from build123d import *

# Parameters (mm, degrees)
BOSS_EXTRUDE1_DEPTH = 63.2
FILLET1_R           = 10
FILLET2_R           = 10
FILLET3_R           = 10
CUT_EXTRUDE1_REACH  = 139.674
SKETCH2_R           = 2.3
SKETCH3_R           = 1.75
CUT_EXTRUDE2_DEPTH  = 138.67396268
SKETCH4_R           = 3.25
CUT_EXTRUDE3_DEPTH  = 7


with BuildPart() as part:
    # Sketch1 → Boss-Extrude1 (new body)
    with BuildSketch(Plane.XY):
        Polygon((114.8, 0), (114.8, 22.5), (92.3, 22.5), (74.008186766, 22.5), (74.008186766, 26), (40.791813234, 26), (40.791813234, 22.5), (22.5, 22.5), (0, 22.5), (0, 0), (0, -16.2), (5, -16.2), (5, 0), (5, 17.5), (22.5, 17.5), (45.791813234, 17.5), (45.791813234, 21), (57.4, 21), (69.008186766, 21), (69.008186766, 17.5), (92.3, 17.5), (109.8, 17.5), (109.8, 0), (109.8, -16.2), (114.8, -16.2), align=None)
    extrude(amount=BOSS_EXTRUDE1_DEPTH)

    # Fillet1
    fillet1_edges = [part.edges().sort_by_distance(p)[0] for p in [
        (0, 22.5, 31.6),
        (114.8, 22.5, 31.6),
        (109.8, 17.5, 31.6),
        (5, 17.5, 31.6),
    ]]
    fillet(fillet1_edges, radius=FILLET1_R)

    # Fillet2
    # the kernel refuses this fillet: 10 mm, written as the material it takes off along each edge
    with BuildSketch(Plane(origin=(40.791813234, 26, -18.998355192), x_dir=(1, 0, 0), z_dir=(0, 0, 1))) as fillet2_piece_1:
        with BuildLine():
            CenterArc((7.599342077, -10), FILLET2_R, 90, 49.458398126)
            Line((0, -3.5), (-0.151986842, -3.37))
            ThreePointArc((-0.151986842, -3.37), (-0.2, -1.75), (-0.2, 0))
            Line((-0.2, 0), (0, 0.2))
            Line((0, 0.2), (7.599342077, 0.2))
            Line((7.599342077, 0.2), (7.599342077, 0))
        make_face()
    extrude(amount=101.196710384, mode=Mode.SUBTRACT)
    with BuildSketch(Plane(origin=(74.008186766, 26, -18.998355192), x_dir=(0, -1, 0), z_dir=(0, 0, 1))) as fillet2_piece_2:
        with BuildLine():
            CenterArc((10, -7.599342077), FILLET2_R, 130.541601874, 49.458398126)
            Line((0, -7.599342077), (-0.2, -7.599342077))
            Line((-0.2, -7.599342077), (-0.2, 0))
            Line((-0.2, 0), (0, 0.2))
            ThreePointArc((0, 0.2), (1.75, 0.2), (3.37, 0.151986842))
            Line((3.37, 0.151986842), (3.5, 0))
        make_face()
    extrude(amount=101.196710384, mode=Mode.SUBTRACT)

    # Fillet3
    # the kernel refuses this fillet: 10 mm, written as the material it takes off along each edge
    with BuildSketch(Plane(origin=(45.791813234, 17.5, -18.998355192), x_dir=(0, 1, 0), z_dir=(0, 0, 1))) as fillet3_piece_1:
        with BuildLine():
            CenterArc((10, 7.599342077), FILLET3_R, 180, 49.458398126)
            Line((0, 7.599342077), (-0.2, 7.599342077))
            Line((-0.2, 7.599342077), (-0.2, 0))
            Line((-0.2, 0), (0, -0.2))
            ThreePointArc((0, -0.2), (1.75, -0.2), (3.37, -0.151986842))
            Line((3.37, -0.151986842), (3.5, 0))
        make_face()
    extrude(amount=101.196710384, mode=Mode.SUBTRACT)
    with BuildSketch(Plane(origin=(69.008186766, 17.5, -18.998355192), x_dir=(1, 0, 0), z_dir=(0, 0, 1))) as fillet3_piece_2:
        with BuildLine():
            CenterArc((7.599342077, 10), FILLET3_R, 220.541601874, 49.458398126)
            Line((0, 3.5), (-0.151986842, 3.37))
            ThreePointArc((-0.151986842, 3.37), (-0.2, 1.75), (-0.2, 0))
            Line((-0.2, 0), (0, -0.2))
            Line((0, -0.2), (7.599342077, -0.2))
            Line((7.599342077, -0.2), (7.599342077, 0))
        make_face()
    extrude(amount=101.196710384, mode=Mode.SUBTRACT)

    # Sketch2 → Cut-Extrude1 (cut, up to next)
    with BuildSketch(Plane(origin=(0, 26, 0), x_dir=(1, 0, 0), z_dir=(0, 1, 0)), mode=Mode.PRIVATE) as cut_extrude1_sk1:
        with Locations(Location((57.4, -9.964206912, 0), (0, 0, 270))):
            Circle(SKETCH2_R)
    cut_extrude1_tool1 = extrude(cut_extrude1_sk1.sketch, amount=-CUT_EXTRUDE1_REACH, mode=Mode.PRIVATE) & part.part
    # Sketch2 → Cut-Extrude1 (cut, up to next)
    with BuildSketch(Plane(origin=(0, 26, 0), x_dir=(1, 0, 0), z_dir=(0, 1, 0)), mode=Mode.PRIVATE) as cut_extrude1_sk2:
        with Locations(Location((57.4, -33.2, 0), (0, 0, 270))):
            Circle(SKETCH2_R)
    cut_extrude1_tool2 = extrude(cut_extrude1_sk2.sketch, amount=-CUT_EXTRUDE1_REACH, mode=Mode.PRIVATE) & part.part
    # Sketch2 → Cut-Extrude1 (cut, up to next)
    with BuildSketch(Plane(origin=(0, 26, 0), x_dir=(1, 0, 0), z_dir=(0, 1, 0)), mode=Mode.PRIVATE) as cut_extrude1_sk3:
        with Locations(Location((57.4, -53.2, 0), (0, 0, 270))):
            Circle(SKETCH2_R)
    cut_extrude1_tool3 = extrude(cut_extrude1_sk3.sketch, amount=-CUT_EXTRUDE1_REACH, mode=Mode.PRIVATE) & part.part
    # Sketch2 → Cut-Extrude1 (cut, up to next)
    with BuildSketch(Plane(origin=(0, 26, 0), x_dir=(1, 0, 0), z_dir=(0, 1, 0)), mode=Mode.PRIVATE) as cut_extrude1_sk4:
        with Locations(Location((21.5, -10, 0), (0, 0, 270))):
            Circle(SKETCH2_R)
    cut_extrude1_tool4 = extrude(cut_extrude1_sk4.sketch, amount=-CUT_EXTRUDE1_REACH, mode=Mode.PRIVATE) & part.part
    # Sketch2 → Cut-Extrude1 (cut, up to next)
    with BuildSketch(Plane(origin=(0, 26, 0), x_dir=(1, 0, 0), z_dir=(0, 1, 0)), mode=Mode.PRIVATE) as cut_extrude1_sk5:
        with Locations(Location((93.3, -9.964206912, 0), (0, 0, 270))):
            Circle(SKETCH2_R)
    cut_extrude1_tool5 = extrude(cut_extrude1_sk5.sketch, amount=-CUT_EXTRUDE1_REACH, mode=Mode.PRIVATE) & part.part
    # Sketch2 → Cut-Extrude1 (cut, up to next)
    with BuildSketch(Plane(origin=(0, 26, 0), x_dir=(1, 0, 0), z_dir=(0, 1, 0)), mode=Mode.PRIVATE) as cut_extrude1_sk6:
        with Locations(Location((93.3, -33.2, 0), (0, 0, 270))):
            Circle(SKETCH2_R)
    cut_extrude1_tool6 = extrude(cut_extrude1_sk6.sketch, amount=-CUT_EXTRUDE1_REACH, mode=Mode.PRIVATE) & part.part
    # Sketch2 → Cut-Extrude1 (cut, up to next)
    with BuildSketch(Plane(origin=(0, 26, 0), x_dir=(1, 0, 0), z_dir=(0, 1, 0)), mode=Mode.PRIVATE) as cut_extrude1_sk7:
        with Locations(Location((93.3, -53.2, 0), (0, 0, 270))):
            Circle(SKETCH2_R)
    cut_extrude1_tool7 = extrude(cut_extrude1_sk7.sketch, amount=-CUT_EXTRUDE1_REACH, mode=Mode.PRIVATE) & part.part
    # Sketch2 → Cut-Extrude1 (cut, up to next)
    with BuildSketch(Plane(origin=(0, 26, 0), x_dir=(1, 0, 0), z_dir=(0, 1, 0)), mode=Mode.PRIVATE) as cut_extrude1_sk8:
        with Locations(Location((21.5, -53.2, 0), (0, 0, 270))):
            Circle(SKETCH2_R)
    cut_extrude1_tool8 = extrude(cut_extrude1_sk8.sketch, amount=-CUT_EXTRUDE1_REACH, mode=Mode.PRIVATE) & part.part
    # Sketch2 → Cut-Extrude1 (cut, up to next)
    with BuildSketch(Plane(origin=(0, 26, 0), x_dir=(1, 0, 0), z_dir=(0, 1, 0)), mode=Mode.PRIVATE) as cut_extrude1_sk9:
        with Locations(Location((21.5, -33.2, 0), (0, 0, 270))):
            Circle(SKETCH2_R)
    cut_extrude1_tool9 = extrude(cut_extrude1_sk9.sketch, amount=-CUT_EXTRUDE1_REACH, mode=Mode.PRIVATE) & part.part
    add(cut_extrude1_tool1.solids().sort_by_distance((57.4, 26, 9.964207))[0], mode=Mode.SUBTRACT)
    add(cut_extrude1_tool2.solids().sort_by_distance((57.4, 26, 33.2))[0], mode=Mode.SUBTRACT)
    add(cut_extrude1_tool3.solids().sort_by_distance((57.4, 26, 53.2))[0], mode=Mode.SUBTRACT)
    add(cut_extrude1_tool4.solids().sort_by_distance((21.5, 26, 10))[0], mode=Mode.SUBTRACT)
    add(cut_extrude1_tool5.solids().sort_by_distance((93.3, 26, 9.964207))[0], mode=Mode.SUBTRACT)
    add(cut_extrude1_tool6.solids().sort_by_distance((93.3, 26, 33.2))[0], mode=Mode.SUBTRACT)
    add(cut_extrude1_tool7.solids().sort_by_distance((93.3, 26, 53.2))[0], mode=Mode.SUBTRACT)
    add(cut_extrude1_tool8.solids().sort_by_distance((21.5, 26, 53.2))[0], mode=Mode.SUBTRACT)
    add(cut_extrude1_tool9.solids().sort_by_distance((21.5, 26, 33.2))[0], mode=Mode.SUBTRACT)

    # Sketch3 → Cut-Extrude2 (cut, through all)
    with BuildSketch(Plane.XZ.offset(16.2)):
        with Locations((2.5, 31.6)):
            Circle(SKETCH3_R)
        with Locations((2.5, 53.6)):
            Circle(SKETCH3_R)
        with Locations((2.5, 9.6)):
            Circle(SKETCH3_R)
        with Locations((112.3, 9.6)):
            Circle(SKETCH3_R)
        with Locations((112.3, 53.6)):
            Circle(SKETCH3_R)
        with Locations((112.3, 31.6)):
            Circle(SKETCH3_R)
    extrude(amount=-CUT_EXTRUDE2_DEPTH, mode=Mode.SUBTRACT)

    # Sketch4 → Cut-Extrude3 (cut)
    with BuildSketch(Plane(origin=(0, 22.5, 0), x_dir=(1, 0, 0), z_dir=(0, 1, 0))):
        with Locations((2.5, -9.6)):
            Circle(SKETCH4_R)
        with Locations((2.5, -31.6)):
            Circle(SKETCH4_R)
        with Locations((2.5, -53.6)):
            Circle(SKETCH4_R)
        with Locations((112.3, -53.6)):
            Circle(SKETCH4_R)
        with Locations((112.3, -31.6)):
            Circle(SKETCH4_R)
        with Locations((112.3, -9.6)):
            Circle(SKETCH4_R)
    extrude(amount=-CUT_EXTRUDE3_DEPTH, mode=Mode.SUBTRACT)


solid = part.part
Read the model definition and answer for the solid it produces. Units are mm, in the model's axes. A direction names the side the tool comes from. Give positions to 0.01 mm unless a question says otherwise; leave off trailing zeros. Write each loop counter-clockwise with the first axis right and the second up, starting at its lowest first coordinate (ties: lowest second). Pieces come first, ordered by that corner, then holes. Notation, with made-up numbers: (37.5, -9) -> (89.5, -9) arc R33 ccw to (89.5, 21) -> close; hole circle Ø6 at (88.25, 49). An arc over 180 degrees is marked (long way). Answer as a JSON object with one key per item and string values. Group by question number.
1) Consider L1, parallel to Z at x = 112, y = 2; L2, parallel to Z at x = 2.5, y = 18.5; L3, parallel to X at y = -3.5, z = 19.5. Determine where each line is inside the solid, lowest interval first. Write a range as from..to.
2) Each of these flat-tipped pins is pushed along its axis until it touches: P1, Ø2.5, axis at x = 111.5, z = 30.5, coming from the +Y side; P2, Ø5.5, axis at x = 93.3, z = 9.96, coming from the -Y side; P3, Ø5, axis at x = 33, z = 53, coming from the +Y side. Where does it stop, or does it pass through?
3) Find section D-D (x = 2.5). Write down the section's boundary in (y, z), and give its area (3 significant figures).
4) Find section B-B (x = 93.3). Write down the section's boundary in (y, z), and give its area (3 significant figures).
5) A tool of negligible diameter and unlimited length cuts with its end or side. For faces 1 (the cylindrical face through (109.05, 17.9, 53.5)), 2 (the cylindrical face through (106.79, 14.65, 32.04)), 3 (the flat face through (57, 22, 0)), from which of +Z, -Z, +X, -X, +Y, -Y can it reach the whole face along a straight path? Write none if from no direction.
6) The mould has two halves that part along X. Classify faces 4 (the flat face through (0, -2, 31)), 5 (the flat face through (90, 22.5, 31)), 6 (the cylindrical face through (72.369, 18.442, 31.158)): +X half, -X half, draft (parallel to the pull), parting line (faces both ways), or undercut.
7) Find section C-C (z = 23). Write down the section's boundary in (x, y).
8) Find section A-A (y = 3). Write down the section's boundary in (x, z).
Values follow:
{
 "1": {"L1": "z = 0..7.88, 11.32..29.88, 33.32..51.88, 55.32..63.2", "L2": "z = 0..6.35, 12.85..28.35, 34.85..50.35, 56.85..63.2", "L3": "x = 0..5, 109.8..114.8"},
 "2": {"P1": "stops at y = 15.5", "P2": "stops at y = 17.5", "P3": "stops at y = 22.5"},
 "3": {"outline": "(-16.2, 0) -> (19.11, 0) -> (19.11, 6.35) -> (15.5, 6.35) -> (15.5, 7.85) -> (-16.2, 7.85) -> close; (-16.2, 11.35) -> (15.5, 11.35) -> (15.5, 12.85) -> (19.11, 12.85) -> (19.11, 28.35) -> (15.5, 28.35) -> (15.5, 29.85) -> (-16.2, 29.85) -> close; (-16.2, 33.35) -> (15.5, 33.35) -> (15.5, 34.85) -> (19.11, 34.85) -> (19.11, 50.35) -> (15.5, 50.35) -> (15.5, 51.85) -> (-16.2, 51.85) -> close; (-16.2, 55.35) -> (15.5, 55.35) -> (15.5, 56.85) -> (19.11, 56.85) -> (19.11, 63.2) -> (-16.2, 63.2) -> close", "area": "1,830 mm2"},
 "4": {"outline": "(17.5, 0) -> (22.5, 0) -> (22.5, 7.66) -> (17.5, 7.66) -> close; (17.5, 12.26) -> (22.5, 12.26) -> (22.5, 30.9) -> (17.5, 30.9) -> close; (17.5, 35.5) -> (22.5, 35.5) -> (22.5, 50.9) -> (17.5, 50.9) -> close; (17.5, 55.5) -> (22.5, 55.5) -> (22.5, 63.2) -> (17.5, 63.2) -> close", "area": "247 mm2"},
 "5": {"face 1": "+Y", "face 2": "+Z, -Z, -Y", "face 3": "-Z, +X, -X, +Y, -Y"},
 "6": {"face 4": "-X half", "face 5": "draft", "face 6": "undercut"},
 "7": {"outline": "(0, -16.2) -> (5, -16.2) -> (5, 7.5) arc R10 cw to (15, 17.5) -> (38.19, 17.5) arc R10 ccw to (45.79, 21) -> (69.01, 21) arc R10 ccw to (76.61, 17.5) -> (99.8, 17.5) arc R10 cw to (109.8, 7.5) -> (109.8, -16.2) -> (114.8, -16.2) -> (114.8, 12.5) arc R10 ccw to (104.8, 22.5) -> (74.01, 22.5) arc R10 ccw to (66.41, 26) -> (48.39, 26) arc R10 ccw to (40.79, 22.5) -> (10, 22.5) arc R10 ccw to (0, 12.5) -> close"},
 "8": {"outline": "(0, 0) -> (5, 0) -> (5, 63.2) -> (0, 63.2) -> close; (109.8, 0) -> (114.8, 0) -> (114.8, 63.2) -> (109.8, 63.2) -> close; hole circle Ø3.5 at (2.5, 9.6); hole circle Ø3.5 at (2.5, 31.6); hole circle Ø3.5 at (2.5, 53.6); hole circle Ø3.5 at (112.3, 9.6); hole circle Ø3.5 at (112.3, 31.6); hole circle Ø3.5 at (112.3, 53.6)"}
}
